Source: CAD feature listing. Evaluate the final solid. Frame: model axes, mm. A direction names the side the tool comes from. Coordinates: 2 decimals unless noted, no trailing zeros. Write each loop counter-clockwise with the first axis right and the second up, starting at its lowest first coordinate (ties: lowest second). Pieces come first, ordered by that corner, then holes. Notation, with made-up numbers: (72, 82.5) - (106, 82.5) arc R20 ccw to (106, 121.5) - close; hole circle Ø11 at (-19, 12). An arc over 180 degrees is marked (long way). One line per question, with ' | ' between items. Start each with the question number.
Q1. Cut plane A-A, the plane x = 0. Return loops of the section in (y, z), plus the area to 3 significant figures.
Q2. Line query: line 1 (Z direction, x = 0.75, y = -19.75); line 2 (Z direction, x = -3.75, y = -9.25); line 3 (Y direction, x = -2, z = 0.25). Output: solid intervals per line, ascending.
Q3. Cut plane C-C, the plane y = -20. Return loops of the section in (x, z).
Q4. Access query for faces 5 (the face through (3, -7, -12)), 6 (the face through (-3, -7, 12)), 7 (the face through (3, -7, 12)). Directions: +Z, -Z, +X, -X, +Y, -Y. A direction counts if a zero-diameter tool reaches every point of the face in a straight line with its end or side. Return the directions, or none.
Q5. Draft query along Z for faces 1 (the face through (-1, -7.25, 14)), 2 (the face through (-0.77, -6.62, 13.94)), 3 (the face through (-9.54, -17.74, 3)), 4 (the face through (0, -15, 0)). Return one class per face: +Z half, -Z half, draft (parallel to the pull), parting line (faces both ways), or undercut.
Q6. Contact query for flat-ended pins moving along their axis: P1, Ø1.5, axis at y = -11.5, z = -4.5, coming from the +X side; P2, Ø1, axis at x = -6, z = -2.5, coming from the +Y side; P3, Ø4, axis at x = -4, y = -18, coming from the +Z side; P4, Ø3, axis at x = 0, z = -12.09, coming from the +Y side. Output: stop coordinate, or through.
Q7. Cut plane B-B, the plane z = 0. Return loops of the section in (x, y), plus the area to 3 significant figures.
Q8. Cut plane D-D, the plane z = 4.75. Return loops of the section in (x, y), plus the area to 3 significant figures.
```python
from build123d import *

# Parameters (mm, degrees)
SKETCH2_R                = 10
BOSS_EXTRUDE1_DEPTH      = 30
CUT_EXTRUDE1_START       = -10
SKETCH3_R                = 10
SKETCH3_R_2              = 7.5
CUT_EXTRUDE1_DEPTH       = 10
CUT_EXTRUDE3_DEPTH       = 10
CUT_EXTRUDE3_DEPTH_BACK  = 10
SKETCH5_R                = 2
FILLET2_R                = 10
BOSS_EXTRUDE2_START      = -67.5
SKETCH7_R                = 10
BOSS_EXTRUDE2_DEPTH      = 67.5
SKETCH8_R                = 50
SKETCH8_R_2              = 10
CUT_EXTRUDE6_DEPTH       = 107.770782567
SKETCH9_R                = 7.5
CUT_EXTRUDE7_DEPTH       = 10
CUT_EXTRUDE8_DEPTH       = 10
CUT_EXTRUDE8_DEPTH_BACK  = 10
SKETCH10_R               = 2
CUT_EXTRUDE9_START       = -60
SKETCH11_R               = 10
SKETCH11_R_2             = 7.5
CUT_EXTRUDE9_DEPTH       = 60
CUT_EXTRUDE10_START      = -60
SKETCH12_R               = 7.5
CUT_EXTRUDE10_DEPTH      = 60
CUT_EXTRUDE11_DEPTH      = 60
CUT_EXTRUDE11_DEPTH_BACK = 60
SKETCH14_R               = 8.5
CUT_EXTRUDE12_DEPTH      = 60
CUT_EXTRUDE12_DEPTH_BACK = 60
SKETCH15_W               = 22.666202576
SKETCH15_H               = 2
BOSS_EXTRUDE3_DEPTH      = 3
BOSS_EXTRUDE3_DEPTH_BACK = 3
SKETCH16_W               = 6
SKETCH16_H               = 1.25
SKETCH18_R               = 2
CUT_EXTRUDE13_DEPTH      = 6.5
CUT_EXTRUDE15_DEPTH      = 16.5
CUT_EXTRUDE15_DEPTH_BACK = 16.5
SKETCH19_W               = 29.449673214
SKETCH19_H               = 14.848126233


with BuildPart() as part:
    # Sketch1 → Revolve1 (revolve)
    with BuildSketch(Plane.XY):
        Polygon((50, 25), (0, 25), (0, 22.5), (45, 22.5), (45, -22.5), (0, -22.5), (0, -25), (50, -25), align=None)
    revolve(axis=Axis((0, -25, 0), (0, 1, 0)))

    # Sketch2 → Boss-Extrude1 (add)
    with BuildSketch(Plane(origin=(0, 25, 0), x_dir=(1, 0, 0), z_dir=(0, 1, 0))):
        with Locations(Location((0, 0, 0), (0, 0, 180))):
            Circle(SKETCH2_R)
    extrude(amount=BOSS_EXTRUDE1_DEPTH)

    # Sketch3 → Cut-Extrude1 (cut)
    with BuildSketch(Plane(origin=(0, 55, 0), x_dir=(1, 0, 0), z_dir=(0, 1, 0)).offset(CUT_EXTRUDE1_START)):
        with Locations(Location((0, 0, 0), (0, 0, 180))):
            Circle(SKETCH3_R)
        with Locations(Location((0, 0, 0), (0, 0, 180))):
            Circle(SKETCH3_R_2, mode=Mode.SUBTRACT)
    extrude(amount=CUT_EXTRUDE1_DEPTH, mode=Mode.SUBTRACT)

    # Sketch5 → Cut-Extrude3 (cut, two sides: drawn at the far end of the back side and taken through both)
    with BuildSketch(Plane(origin=(0, 0, 0), x_dir=(0, 0, -1), z_dir=(1, 0, 0)).offset(-CUT_EXTRUDE3_DEPTH_BACK)):
        with Locations(Location((0, 50, 0), (0, 0, 180))):
            Circle(SKETCH5_R)
    extrude(amount=CUT_EXTRUDE3_DEPTH + CUT_EXTRUDE3_DEPTH_BACK, mode=Mode.SUBTRACT)

    # Fillet2
    fillet2_edges = [part.edges().sort_by_distance(p)[0] for p in [
        (-50, 25, 0),
    ]]
    fillet(fillet2_edges, radius=FILLET2_R)

    # Sketch7 → Boss-Extrude2 (add)
    with BuildSketch(Plane(origin=(0, 45, 0), x_dir=(1, 0, 0), z_dir=(0, 1, 0)).offset(BOSS_EXTRUDE2_START)):
        with Locations(Location((0, 0, 0), (0, 0, 180))):
            Circle(SKETCH7_R)
    extrude(amount=BOSS_EXTRUDE2_DEPTH)

    # Sketch8 → Cut-Extrude6 (cut, through all)
    with BuildSketch(Plane(origin=(0, 55, 0), x_dir=(1, 0, 0), z_dir=(0, 1, 0))):
        Circle(SKETCH8_R)
        with Locations(Location((0, 0, 0), (0, 0, 180))):
            Circle(SKETCH8_R_2, mode=Mode.SUBTRACT)
    extrude(amount=-CUT_EXTRUDE6_DEPTH, mode=Mode.SUBTRACT)

    # Sketch9 → Cut-Extrude7 (cut)
    with BuildSketch(Plane.XZ.offset(25)):
        with Locations(Location((0, 0, 0), (0, 0, 180))):
            Circle(SKETCH9_R)
    extrude(amount=-CUT_EXTRUDE7_DEPTH, mode=Mode.SUBTRACT)

    # Sketch10 → Cut-Extrude8 (cut, two sides: drawn at the far end of the back side and taken through both)
    with BuildSketch(Plane(origin=(0, 0, 0), x_dir=(0, 0, -1), z_dir=(1, 0, 0)).offset(-CUT_EXTRUDE8_DEPTH_BACK)):
        with Locations(Location((0, -20, 0), (0, 0, 180))):
            Circle(SKETCH10_R)
    extrude(amount=CUT_EXTRUDE8_DEPTH + CUT_EXTRUDE8_DEPTH_BACK, mode=Mode.SUBTRACT)

    # Sketch11 → Cut-Extrude9 (cut)
    with BuildSketch(Plane(origin=(0, 55, 0), x_dir=(1, 0, 0), z_dir=(0, 1, 0)).offset(CUT_EXTRUDE9_START)):
        with Locations(Location((0, 0, 0), (0, 0, 180))):
            Circle(SKETCH11_R)
        Circle(SKETCH11_R_2, mode=Mode.SUBTRACT)
    extrude(amount=CUT_EXTRUDE9_DEPTH, mode=Mode.SUBTRACT)

    # Sketch12 → Cut-Extrude10 (cut)
    with BuildSketch(Plane(origin=(0, 55, 0), x_dir=(1, 0, 0), z_dir=(0, 1, 0)).offset(CUT_EXTRUDE10_START)):
        Circle(SKETCH12_R)
    extrude(amount=CUT_EXTRUDE10_DEPTH, mode=Mode.SUBTRACT)

    # Sketch13 → Revolve2 (revolve)
    with BuildSketch(Plane(origin=(0, 0, 0), x_dir=(0, 0, -1), z_dir=(1, 0, 0))):
        with BuildLine():
            Line((0, -15), (0, 5))
            ThreePointArc((0, 5), (-10, -5), (0, -15))
        make_face()
    revolve(axis=Axis((0, -15, 0), (0, 1, 0)))

    # Sketch14 → Cut-Extrude11 (cut, two sides: drawn at the far end of the back side and taken through both)
    with BuildSketch(Plane(origin=(0, 0, 0), x_dir=(0, 0, -1), z_dir=(1, 0, 0)).offset(-CUT_EXTRUDE11_DEPTH_BACK)):
        with Locations(Location((0, -5, 0), (0, 0, 180))):
            Circle(SKETCH14_R)
    extrude(amount=CUT_EXTRUDE11_DEPTH + CUT_EXTRUDE11_DEPTH_BACK, mode=Mode.SUBTRACT)

    # Sketch15 → Cut-Extrude12 (cut, two sides: drawn at the far end of the back side and taken through both)
    with BuildSketch(Plane(origin=(0, 0, 0), x_dir=(0, 0, -1), z_dir=(1, 0, 0)).offset(-CUT_EXTRUDE12_DEPTH_BACK)):
        with Locations((0, -5)):
            Rectangle(SKETCH15_W, SKETCH15_H)
    extrude(amount=CUT_EXTRUDE12_DEPTH + CUT_EXTRUDE12_DEPTH_BACK, mode=Mode.SUBTRACT)


with BuildPart() as cut_extrude12_piece_1:
    # of the separate pieces the step leaves, piece 1, a body of its own (cut_extrude12_pieces)
    add(part.part.solids().sort_by_distance((-10, -25, 0))[0])



with BuildPart() as cut_extrude12_piece_2:
    # of the separate pieces the step leaves, piece 2, a body of its own (cut_extrude12_pieces)
    add(part.part.solids().sort_by_distance((5.267826876, -4, 8.440971508))[0])


with BuildPart() as cut_extrude12_piece_1_1:
    add(cut_extrude12_piece_1.part)

    add(cut_extrude12_piece_2.part)  # Boss-Extrude3 merges Cut-Extrude12 piece 2
    # Sketch16 → Boss-Extrude3 (add, two sides: drawn at the far end of the back side and taken through both)
    with BuildSketch(Plane(origin=(0, 0, 0), x_dir=(0, 0, -1), z_dir=(1, 0, 0)).offset(-BOSS_EXTRUDE3_DEPTH_BACK)):
        with Locations((-11.440971508, -3.375)):
            Rectangle(SKETCH16_W, SKETCH16_H)
        with Locations((11.440971508, -3.375)):
            Rectangle(SKETCH16_W, SKETCH16_H)
        with Locations((11.440971508, -6.625)):
            Rectangle(SKETCH16_W, SKETCH16_H)
        with Locations((-11.440971508, -6.625)):
            Rectangle(SKETCH16_W, SKETCH16_H)
    extrude(amount=BOSS_EXTRUDE3_DEPTH + BOSS_EXTRUDE3_DEPTH_BACK)

    # Sketch18 → Cut-Extrude13 (cut)
    with BuildSketch(Plane(origin=(0, -2.75, 0), x_dir=(1, 0, 0), z_dir=(0, 1, 0))):
        with Locations(Location((0, 12.092279572, 0), (0, 0, 270))):
            Circle(SKETCH18_R)
        with Locations(Location((0, -12.092279572, 0), (0, 0, 270))):
            Circle(SKETCH18_R)
    extrude(amount=-CUT_EXTRUDE13_DEPTH, mode=Mode.SUBTRACT)

    # Sketch19 → Cut-Extrude15 (cut, two sides: drawn at the far end of the back side and taken through both)
    with BuildSketch(Plane(origin=(0, 0, 0), x_dir=(0, 0, -1), z_dir=(1, 0, 0)).offset(-CUT_EXTRUDE15_DEPTH_BACK)):
        with Locations((-0.022434936, 1.737788606)):
            Rectangle(SKETCH19_W, SKETCH19_H)
    extrude(amount=CUT_EXTRUDE15_DEPTH + CUT_EXTRUDE15_DEPTH_BACK, mode=Mode.SUBTRACT)


solid = cut_extrude12_piece_1_1.part
```
Reply:
1) outline: (-25, -10) - (-7.25, -10) - (-7.25, -10.09) - (-6, -10.09) - (-6, -8.44) arc R8.5 cw to (-6, 8.44) - (-6, 10.09) - (-7.25, 10.09) - (-7.25, 10) - (-25, 10) - (-25, 7.5) - (-15, 7.5) - (-15, -7.5) - (-25, -7.5) - close; (-7.25, -14.44) - (-6, -14.44) - (-6, -14.09) - (-7.25, -14.09) - close; (-7.25, 14.09) - (-6, 14.09) - (-6, 14.44) - (-7.25, 14.44) - close | area: 135 mm^2
2) line 1: z = -9.97 to -7.46, 7.46 to 9.97 | line 2: z = -9.27 to -7.36, 7.36 to 9.27 | line 3: y = -15 to -13.5
3) outline: (-9.8, -2) arc R10 ccw to (9.8, -2) - (7.23, -2) arc R7.5 cw to (-7.23, -2) - close; (-9.8, 2) - (-7.23, 2) arc R7.5 cw to (7.23, 2) - (9.8, 2) arc R10 ccw to start
4) face 5: -Z, +X, +Y, -Y | face 6: +Z, -X, +Y, -Y | face 7: +Z, +X, +Y, -Y
5) face 1: draft | face 2: undercut | face 3: parting line | face 4: undercut
6) P1: stops at x = 8.96 | P2: stops at y = -12.95 | P3: stops at z = 9.8 | P4: passes through
7) outline: (-10, -25) - (-7.5, -25) - (-7.5, -22) - (-10, -22) - close; (-10, -18) - (-7.5, -18) - (-7.5, -15) - (7.5, -15) - (7.5, -18) - (10, -18) - (10, -13.5) - (-10, -13.5) - close; (7.5, -25) - (10, -25) - (10, -22) - (7.5, -22) - close | area: 60.0 mm^2
8) outline: (-8.8, -25) - (-5.8, -25) - (-5.8, -15) - (5.8, -15) - (5.8, -25) - (8.8, -25) - (8.8, -12.05) - (-8.8, -12.05) - close | area: 112 mm^2
